Verification items for the finished model (mm, model axes). A direction names the side the tool comes from. Give positions to 0.01 mm unless a question says otherwise; leave off trailing zeros. Loops run counter-clockwise (first coordinate to the right, second up) from the corner with the lowest first, then second, coordinate; pieces in that order, holes last. Notation, with made-up numbers: (42.25, 8.5) - (77.25, 8.5) arc R31 ccw to (77.25, 34.5) - close; hole circle Ø4 at (3, 63). An arc over 180 degrees is marked (long way). Answer in a Markdown table with one row per item.
Solid Edge part; units mm, degrees
sketch "Sketch1" plane through (0, 0, 0) normal (0, 0, 1) x (1, 0, 0)
  circle A0 centre (0, 0) radius 19.05
extrude "Protrusion1" add sketch "Sketch1" against normal blind 82.55
sketch "Sketch2" plane through (0, 0, 0) normal (0, 0, 1) x (1, 0, 0)
  line L0 (-22.225, -9.2059) -> (-9.2059, -22.225)
  line L1 (-9.2059, -22.225) -> (9.2059, -22.225)
  line L2 (9.2059, -22.225) -> (22.225, -9.2059)
  line L3 (22.225, -9.2059) -> (22.225, 9.2059)
  line L4 (22.225, 9.2059) -> (9.2059, 22.225)
  line L5 (9.2059, 22.225) -> (-9.2059, 22.225)
  line L6 (-9.2059, 22.225) -> (-22.225, 9.2059)
  line L7 (-22.225, 9.2059) -> (-22.225, -9.2059)
extrude "ExtrudedProtrusion_2" add sketch "Sketch2" along normal blind 12.7
chamfer "Chamfer_1" distance 3.1826 angle 45 8 edges at (15.7154, -15.7154, 12.7) (22.225, 0, 12.7) (15.7154, 15.7154, 12.7) (0, 22.225, 12.7) (-15.7154, 15.7154, 12.7) (-22.225, 0, 12.7) (-15.7154, -15.7154, 12.7) (0, -22.225, 12.7)
Q1. Sectioned sample at C-C (z = -63.5). Record the cut outline in (x, y).
Completed:
| item | result |
|---|---|
| outline | circle Ø38.1 at (0, 0) |
Q2. Thickness scan on line 1 (Y direction, x = 1, z = -41); line 2 (Y direction, x = 13, z = -55); line 3 (Z direction, x = 13, y = -14). Record the ranges inside material, lowest first.
Completed:
| item | result |
|---|---|
| line 1 | -19.02 to 19.02 |
| line 2 | -13.92 to 13.92 |
| line 3 | 0 to 12.65 |
Q3. Go/stop test with flat-tipped pins: P1, Ø1, axis at x = 14, y = -15, coming from the +Z side; P2, Ø5, axis at x = 13.5, z = -23, coming from the -Y side; P3, Ø6, axis at x = -7, z = -36.5, coming from the -Y side. Record where each tip stops, or that it passes through.
Completed:
| item | result |
|---|---|
| P1 | z = 11.74 |
| P2 | y = -15.55 |
| P3 | y = -18.63 |
Q4. Tool access check on faces 1 (the face through (15.81, 15.62, 4.69)), 2 (the face through (-15.12, -11.59, -40.7)). Record the directions out of +Z, -Z, +X, -X, +Y, -Y that give a thin tool (end or side, any length) a straight path to the whole face; none if there is none.
Completed:
| item | result |
|---|---|
| face 1 | +Z, -Z, +X, +Y |
| face 2 | -Z |
Q5. Sectioned sample at A-A (x = 0). Record the cut outline in (y, z) (3 decimals).
Completed:
| item | result |
|---|---|
| outline | (-22.225, 0) - (-19.05, 0) - (-19.05, -82.55) - (19.05, -82.55) - (19.05, 0) - (22.225, 0) - (22.225, 9.517) - (19.042, 12.7) - (-19.042, 12.7) - (-22.225, 9.517) - close |
